CAD build for the part. Positions are in the model's coordinates, mm. Face numbers are marked on the shaded views. A direction names the side the tool comes from. Round coordinates to 2 decimals unless told otherwise and drop trailing zeros. Write each loop counter-clockwise with the first axis right and the second up, starting at its lowest first coordinate (ties: lowest second). Pieces come first, ordered by that corner, then holes. Notation, with made-up numbers: M -8,81 L 47,81 A16 cw 47,100 Z; hole C 3,9 d7. An arc over 180 degrees is marked long. Write each question's results on one line, items separated by ' | '. Start each with the question number.
```python
from build123d import *

# Parameters (mm, degrees)
ESBO_O1_W                = 42.3
ESBO_O1_H                = 42.3
RESSALTO_EXTRUS_O1_DEPTH = 21.15
ESBO_O2_R                = 11.025
RESSALTO_EXTRUS_O2_DEPTH = 2
CHANFRO1_SIZE            = 5.6
ESBO_O4_R                = 1.65
CORTE_EXTRUS_O1_DEPTH    = 10
ESBO_O3_R                = 4
CORTE_EXTRUS_O2_DEPTH    = 70


with BuildPart() as part:
    # Esboço1 → Ressalto-extrusão1 (new body, symmetric)
    with BuildSketch(Plane(origin=(0, 0, 0), x_dir=(1, 0, 0), z_dir=(0, 1, 0))):
        Rectangle(ESBO_O1_W, ESBO_O1_H)
    extrude(amount=RESSALTO_EXTRUS_O1_DEPTH, both=True)

    # Esboço2 → Ressalto-extrusão2 (add)
    with BuildSketch(Plane(origin=(0, 21.15, 0), x_dir=(1, 0, 0), z_dir=(0, 1, 0))):
        Circle(ESBO_O2_R)
    extrude(amount=RESSALTO_EXTRUS_O2_DEPTH)

    # Chanfro1
    chanfro1_edges = [part.edges().sort_by_distance(p)[0] for p in [
        (21.15, 0, 21.15),
        (-21.15, 0, 21.15),
        (-21.15, 0, -21.15),
        (21.15, 0, -21.15),
    ]]
    chamfer(chanfro1_edges, length=CHANFRO1_SIZE)

    # Esboço4 → Corte-extrusão1 (cut)
    with BuildSketch(Plane(origin=(0, 21.15, 0), x_dir=(1, 0, 0), z_dir=(0, 1, 0))):
        with Locations((-15.05, 15.05)):
            Circle(ESBO_O4_R)
        with Locations((15.05, 15.05)):
            Circle(ESBO_O4_R)
        with Locations((15.05, -15.05)):
            Circle(ESBO_O4_R)
        with Locations((-15.05, -15.05)):
            Circle(ESBO_O4_R)
    extrude(amount=-CORTE_EXTRUS_O1_DEPTH, mode=Mode.SUBTRACT)

    # Esboço3 → Corte-extrusão2 (cut)
    with BuildSketch(Plane(origin=(0, 23.15, 0), x_dir=(1, 0, 0), z_dir=(0, 1, 0))):
        Circle(ESBO_O3_R)
    extrude(amount=-CORTE_EXTRUS_O2_DEPTH, mode=Mode.SUBTRACT)


solid = part.part
```
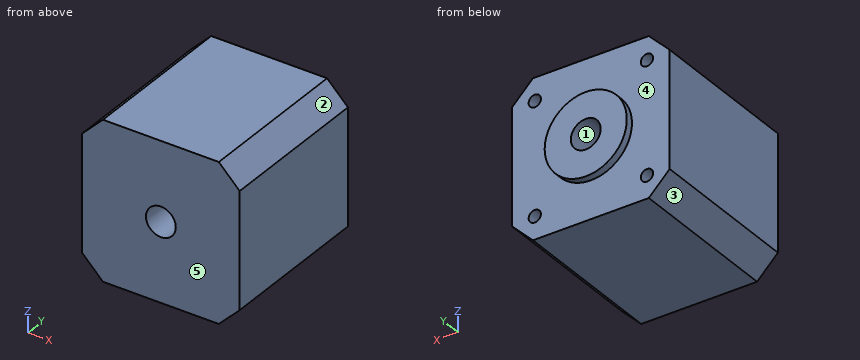
1) Saw through at C-C, the plane x = 3. Write the cut outline in (y, z).
2) Saw through at D-D, the plane y = 13.5. Write the cut outline in (x, z), plus the area to 3 significant figures.
3) 3-axis set-ups, long thin cutter, end or side, ignore diameter. For the marked faces 4 and 5: which of +Z, -Z, +X, -X, +Y, -Y reach the whole face in a straight line?
4) Saw through at A-A, the plane z = 0. Write the cut outline in (x, y) (3 decimals).
5) Wall check: line 1 along X through (y, z) = (16.75, 15.05); line 2 along Y through (x, z) = (-15, 16). Give the ranges that are in metal, low to high. Write a range as from..to.
6) Saw through at B-B, the plane y = -1. Write the cut outline in (x, z), plus the area to 3 significant figures.
7) Pull direction X, two halves, no side cores. Call the marked faces 1, 2 and 3: pulls with the +X half, pulls with the -X half, needs draft (parallel to the pull), parting line crosses it, or undercut.
8) Drop flat-ended pins along their axis: pin 1 Ø2.5 at (x, z) = (-14.5, 14.5) entering from +Y; pin 2 Ø3 at (x, z) = (-15.05, -15.05) entering from +Y. Give the stop position or say it passes through.
Filled sheet:
1) outline: M -21.15,-21.15 L 21.15,-21.15 L 21.15,-10.61 L 23.15,-10.61 L 23.15,-2.65 L -21.15,-2.65 Z; M -21.15,2.65 L 23.15,2.65 L 23.15,10.61 L 21.15,10.61 L 21.15,21.15 L -21.15,21.15 Z
2) outline: M -21.15,-15.55 L -15.55,-21.15 L 15.55,-21.15 L 21.15,-15.55 L 21.15,15.55 L 15.55,21.15 L -15.55,21.15 L -21.15,15.55 Z; hole C -15.05,-15.05 d3.3; hole C -15.05,15.05 d3.3; hole C 0,0 d8; hole C 15.05,-15.05 d3.3; hole C 15.05,15.05 d3.3 | area: 1,640 mm^2
3) face 4: +Y | face 5: +Z, -Z, +X, -X, -Y
4) outline: M -21.15,-21.15 L -4,-21.15 L -4,23.15 L -11.025,23.15 L -11.025,21.15 L -21.15,21.15 Z; M 4,-21.15 L 21.15,-21.15 L 21.15,21.15 L 11.025,21.15 L 11.025,23.15 L 4,23.15 Z
5) line 1: x = -21.15..-16.7, -13.4..13.4, 16.7..21.15 | line 2: y = -21.15..11.15
6) outline: M -21.15,-15.55 L -15.55,-21.15 L 15.55,-21.15 L 21.15,-15.55 L 21.15,15.55 L 15.55,21.15 L -15.55,21.15 L -21.15,15.55 Z; hole C 0,0 d8 | area: 1,680 mm^2
7) face 1: undercut | face 2: pulls with the +X half | face 3: pulls with the -X half
8) pin 1: stops at y = 21.15 | pin 2: stops at y = 11.15
